Model file for the job. Use its own axes, mm. Face numbers are marked on the shaded views. A direction names the side the tool comes from. Round coordinates to 2 decimals unless told otherwise and drop trailing zeros. Loops run counter-clockwise (first coordinate to the right, second up) from the corner with the lowest first, then second, coordinate; pieces in that order, holes last. Notation, with made-up numbers: (34, 11.5) - (54, 11.5) arc R18 cw to (54, 21.5) - close; hole circle Ø7 at (-31.5, 81). An arc over 180 degrees is marked (long way). Use one line per item in the form item = value.
from build123d import *

# Parameters (mm, degrees)
EXTRUSION1_DEPTH        = 20
ENL_V_MAT_EXTRU_1_DEPTH = 62.64414003
ESQUISSE3_R             = 2.25
ENL_V_MAT_EXTRU_2_DEPTH = 62.64414003


with BuildPart() as part:
    # Esquisse1 → Extrusion1 (new body)
    with BuildSketch(Plane.XY):
        with BuildLine():
            Line((0, 0), (0, 50))
            Line((0, 50), (1, 50))
            Line((1, 50), (1, 0))
            ThreePointArc((1, 0), (0.707106781, -0.707106781), (0, -1))
            Line((0, -1), (-30, -1))
            Line((-30, -1), (-30, 0))
            Line((-30, 0), (0, 0))
        make_face()
    extrude(amount=EXTRUSION1_DEPTH)

    # Esquisse2 → Enlèv. mat.-Extru.1 (cut, through all)
    with BuildSketch(Plane.ZY):
        with BuildLine():
            Line((5, 35), (5, 31))
            ThreePointArc((5, 31), (10, 26), (15, 31))
            Line((15, 31), (15, 35))
            ThreePointArc((15, 35), (10, 40), (5, 35))
        make_face()
    extrude(amount=-ENL_V_MAT_EXTRU_1_DEPTH, mode=Mode.SUBTRACT)

    # Esquisse3 → Enlèv. mat.-Extru.2 (cut, through all)
    with BuildSketch(Plane(origin=(0, 0, 0), x_dir=(-1, 0, 0), z_dir=(0, 1, 0))):
        with Locations((10, 10)):
            Circle(ESQUISSE3_R)
        with Locations((20, 10)):
            Circle(ESQUISSE3_R)
    extrude(amount=-ENL_V_MAT_EXTRU_2_DEPTH, mode=Mode.SUBTRACT)


solid = part.part
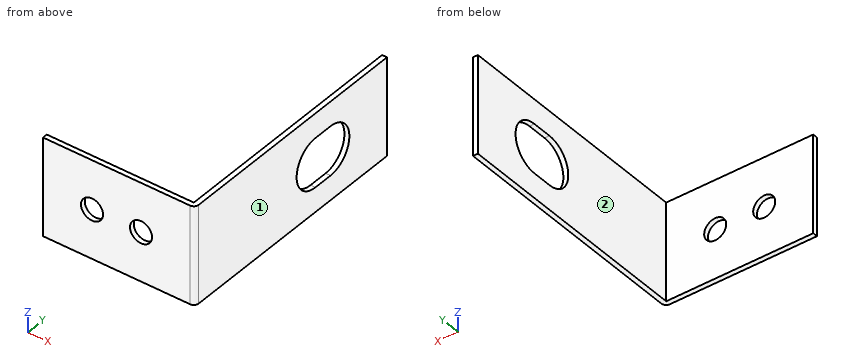
1. Cut at D-D, the plane x = -27. Give the cut face in (y, z).
Geometry check:
outline = (-1, 0) - (0, 0) - (0, 20) - (-1, 20) - close
2. Cut at B-B, the plane z = 2.75. Give the cut face in (x, y), plus the area to 3 significant figures.
Geometry check:
outline = (-30, -1) - (0, -1) arc R1 ccw to (1, 0) - (1, 50) - (0, 50) - (0, 0) - (-30, 0) - close
area = 80.8 mm^2
3. Cut at C-C, the plane y = 20.5. Give the cut face in (x, z), plus the area to 3 significant figures.
Geometry check:
outline = (0, 0) - (1, 0) - (1, 20) - (0, 20) - close
area = 20.0 mm^2
4. Tool access for the marked faces 1 and 2: list every direction of +Z, -Z, +X, -X, +Y, -Y with a clear straight run to the whole face (end or side of a thin tool).
Geometry check:
face_1 = +Z, -Z, +X, +Y, -Y
face_2 = +Z, -Z, -X, +Y
5. Cut at A-A, the plane x = -20. Give the cut face in (y, z).
Geometry check:
outline = (-1, 0) - (0, 0) - (0, 7.75) - (-1, 7.75) - close; (-1, 12.25) - (0, 12.25) - (0, 20) - (-1, 20) - close
6. Wall check: probe 1 along Z at (x, y) = (-20, -0.25); probe 2 along Y at (x, z) = (-6, 15.75); probe 3 along X at (y, z) = (16, 15.25). Give the ranges that are in metal, low to high.
Geometry check:
probe_1 = 0 to 7.75, 12.25 to 20
probe_2 = -1 to 0
probe_3 = 0 to 1
7. Flat gauge pins, fed straight in: pin 1 (6 mm diameter, centred on x = -6.5, z = 7.5, fed in from +Y); pin 2 (10 mm diameter, centred on y = 25.5, z = 17, fed in from -X); pin 3 (1.5 mm diameter, centred on x = -10.5, z = 11, fed in from -Y). Where does each tip first touch, or does it go through?
Geometry check:
pin_1 = 0
pin_2 = 0
pin_3 = through
